Study the drawing (mm; zero at the part's minimum x, y, z) and answer. A direction names the side the tool comes from. Coordinates: 2 decimals unless noted, no trailing zeros. Order: outer loops, then holes, each group sorted by start corner. A loop starts at its lowest first (then second) coordinate and runs counter-clockwise, first axis right, second up.
1. Find the intervals of material crossed by probe 1 along X at (y, z) = (463.5, 274); probe 2 along X at (y, z) = (149, 386.5); probe 3 along Y at (x, z) = (633.5, 244.5), in increasing order.
2. A tool of negligible diameter and unlimited length cuts with its end or side. For the marked faces 4, 5, 6, 7 and 8, from which of +Z, -Z, +X, -X, +Y, -Y can it reach the whole face along a straight path? Write none if from no direction.
3. The part is cut by section B-B, the plane x = 720. Give the vertices of the cut face in (y, z).
4. The part is cut by section D-D, the plane x = 126. Give the vertices of the cut face in (y, z), then the cut area to 3 significant figures.
5. The part is cut by section C-C, the plane z = 242. Give the vertices of the cut face in (x, y), then the cut area to 3 significant figures.
6. The part is cut by section A-A, the plane y = 495. Give the vertices of the cut face in (x, z).
7. Flat-ended cylindrical pins translate along their axes: pin 1 Ø4 at (x, y) = (456, 277.5) entering from +Z; pin 2 Ø2 at (y, z) = (538.5, 254.5) entering from -X; pin 3 Ø25 at (x, y) = (509.5, 123.5) entering from +Z; pin 4 Ø24 at (x, z) = (391.5, 323) entering from +Y. Find the tip coordinate at first contact, or state that the pin passes through.
8. Determine the mould class of the marked faces 1, 2 and 3 for opening direction X: +X half, -X half, draft (parallel to the pull), parting line (faces both ways), or undercut.
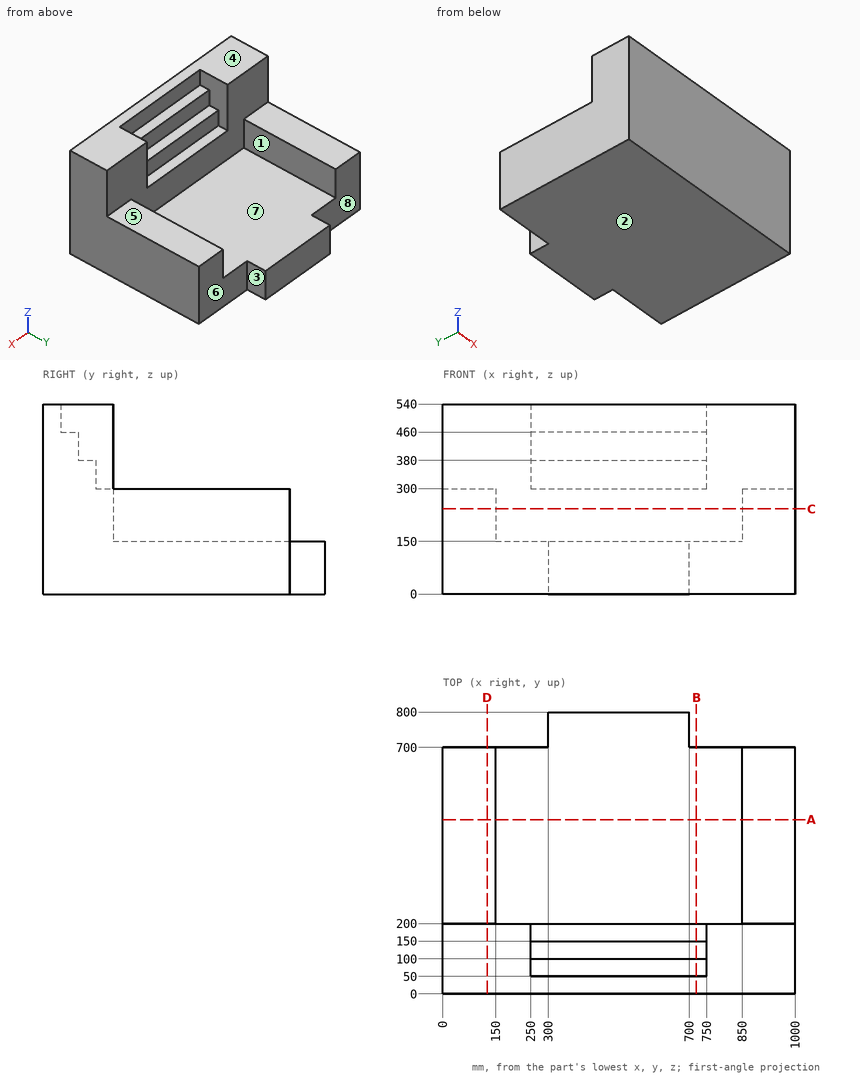
Geometry says:
1. probe 1: x = 0 to 150, 850 to 1000
1. probe 2: x = 0 to 250, 750 to 1000
1. probe 3: y = 0 to 200
2. face 4: +Z, +X, -X, +Y, -Y
2. face 5: +Z, +X, -X, +Y
2. face 6: +Z, -Z, +X, +Y
2. face 7: +Z, +Y
2. face 8: +Z, -Z, -X, +Y
3. outline: (0, 0) - (700, 0) - (700, 150) - (200, 150) - (200, 300) - (150, 300) - (150, 380) - (100, 380) - (100, 460) - (50, 460) - (50, 540) - (0, 540) - close
4. outline: (0, 0) - (700, 0) - (700, 300) - (200, 300) - (200, 540) - (0, 540) - close
4. area: 258,000 mm2
5. outline: (0, 0) - (1000, 0) - (1000, 700) - (850, 700) - (850, 200) - (150, 200) - (150, 700) - (0, 700) - close
5. area: 350,000 mm2
6. outline: (0, 0) - (1000, 0) - (1000, 300) - (850, 300) - (850, 150) - (150, 150) - (150, 300) - (0, 300) - close
7. pin 1: stops at z = 150
7. pin 2: stops at x = 0
7. pin 3: stops at z = 380
7. pin 4: stops at y = 150
8. face 1: undercut
8. face 2: draft
8. face 3: +X half
